```python
from build123d import *

# Parameters (mm, degrees)
F0_W     = 27.3
F0_H     = 27.8
F0_W_2   = 26.67
F0_H_2   = 19.26
F0_W_3   = 22.86
F0_H_3   = 12.7
F1_DEPTH = 1.143
F2_DEPTH = 1.5
F3_DEPTH = 1.51
F5_D     = 2


with BuildPart() as f1:
    # F0 (on Top) → F1 (new body)
    with BuildSketch(Plane.XY):
        with Locations((0, -2.191441)):
            Rectangle(F0_W, F0_H)
        with Locations((0, -2.191441)):
            Rectangle(F0_W_2, F0_H_2, mode=Mode.SUBTRACT)
        with Locations((0, -2.191441)):
            Rectangle(F0_W_2, F0_H_2)
        Rectangle(F0_W_3, F0_H_3, mode=Mode.SUBTRACT)
        Rectangle(F0_W_3, F0_H_3)
    extrude(amount=-F1_DEPTH)

    # F0 (on Top) → F2 (join)
    with BuildSketch(Plane.XY):
        with Locations((0, -2.191441)):
            Rectangle(F0_W_2, F0_H_2)
        Rectangle(F0_W_3, F0_H_3, mode=Mode.SUBTRACT)
        Rectangle(F0_W_3, F0_H_3)
    extrude(amount=F2_DEPTH)

    # F0 (on Top) → F3 (join)
    with BuildSketch(Plane.XY):
        Rectangle(F0_W_3, F0_H_3)
    extrude(amount=F3_DEPTH)

    # F5 (through all)
    with Locations(Plane.XY):
        with Locations((-11.65, 9.708559), (11.65, 9.708559), (11.65, -14.091441), (-11.65, -14.091441)):
            Hole(F5_D / 2)


solid = f1.part
```
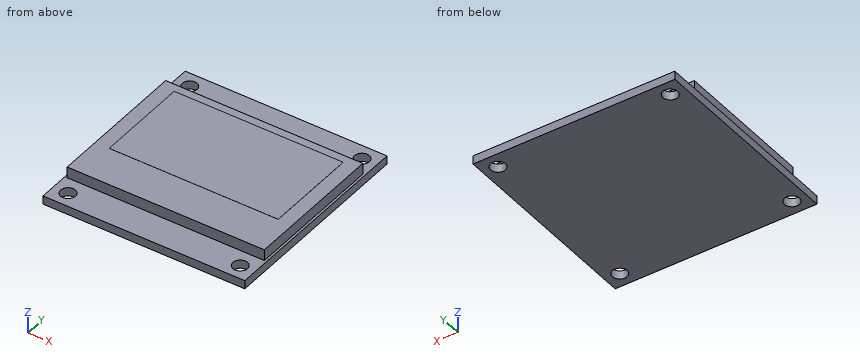
Here's how the part is built. I have some questions about the finished solid (model axes, mm). Round coordinates to 2 decimals unless told otherwise and drop trailing zeros. Order: outer loops, then holes, each group sorted by start corner. A loop starts at its lowest first (then second) coordinate and runs counter-clockwise, first axis right, second up. Notation, with made-up numbers: M -5.75,41 L 11.25,41 A33 ccw 11.25,74 Z; hole C 12,-23.5 d3. An arc over 180 degrees is marked long. Answer as CSV lines item,"result".
Item 1: Please list where these lines run through material, in increasing order: L1, parallel to Y at x = -11.65, z = -0.7; L2, parallel to Z at x = 5, y = -7.25; L3, parallel to Z at x = 10, y = 8.5. Write a range as [from, to].
From the geometry:
L1,"[-16.09, -15.09], [-13.09, 8.71], [10.71, 11.71]"
L2,"[-1.14, 1.5]"
L3,"[-1.14, 0]"
Item 2: Imagine slicing it at C-C on z = 0.5. List the corners of the cut face in (x, y) for me (3 decimals).
From the geometry:
outline,"M -13.335,-11.821 L 13.335,-11.821 L 13.335,7.439 L -13.335,7.439 Z"
Item 3: Imagine slicing it at A-A on y = -7.75. List the corners of the cut face in (x, z) for me (3 decimals).
From the geometry:
outline,"M -13.65,-1.143 L 13.65,-1.143 L 13.65,0 L 13.335,0 L 13.335,1.5 L -13.335,1.5 L -13.335,0 L -13.65,0 Z"
Item 4: For pin 1 (1.8 mm diameter, centred on x = -11.65, y = -14.09, fed in from +Z); pin 2 (0.8 mm diameter, centred on x = -1, z = 0.5, fed in from -Y); pin 3 (1.2 mm diameter, centred on y = -2, z = 1, fed in from +X) (3 decimals); pin 4 (2.5 mm diameter, centred on x = 11.65, y = 9.71, fed in from +Z), each with a flat end and sliding along its axis, tell me the tip position at first contact or that it passes through.
From the geometry:
pin 1,"through"
pin 2,"y = -11.82"
pin 3,"x = 13.335"
pin 4,"z = 0"
